Check sheet for the modelled part. Datum: model origin and axes. Units: mm. A direction names the side the tool comes from. Round coordinates to 2 decimals unless told otherwise and drop trailing zeros. Order: outer loops, then holes, each group sorted by start corner. A loop starts at its lowest first (then second) coordinate and runs counter-clockwise, first axis right, second up.
Q1. Set-up check for faces 1 (the flat face through (140, 20, -29.5)), 2 (the flat face through (66.49, 8.03, -16.82)), 3 (the flat face through (66.04, 12.08, -16.82)): record each of +Z, -Z, +X, -X, +Y, -Y from which the full face is reachable in a straight line by a thin tool's end or side.
Q2. Cross-section at A-A on x = 16.5. Record the cut outline in (y, z), then the cut area to 3 significant figures.
Q3. Depth check by flat-ended pin: P1, Ø8, axis at x = 133, y = 16, coming from the +Z side; P2, Ø10, axis at x = 160.5, z = -3.5, coming from the -Y side; P3, Ø4.5, axis at x = 246.5, z = -17, coming from the -Y side; P4, Ø3, axis at x = 235.5, z = -4, coming from the +Y side. Enter the tip coordinate at first touch or a pass-through.
Q4. Mould release check, pull along Z, two halves, no side actions. Record for faces 4 (the flat face through (250, 5, -34)), 5 (the cylindrical face through (16.6, 3.5, -19.5)), 6 (the flat face through (214.4, 11.944, -16.825)): +Z half, -Z half, draft (parallel to the pull), parting line (faces both ways), or undercut.
Q5. Cross-section at B-B on x = 213. Record the cut outline in (y, z).
Q6. Scan lines: probe 1 along X at (y, z) = (1.5, -17); probe 2 along X at (y, z) = (3, -16); probe 3 along Y at (x, z) = (18.5, -9.5). Record each from-to range of solid material in increasing order.
from build123d import *

# Parameters (mm, degrees)
SKETCH1_W             = 50
SKETCH1_H             = 34
BOSS_EXTRUDE1_DEPTH   = 10
BOSS_EXTRUDE1_2_DEPTH = 10
FILLET1_R             = 10
FILLET2_R             = 10
BOSS_EXTRUDE2_DEPTH   = 12.5
SKETCH4_R             = 2.5
CUT_EXTRUDE1_DEPTH    = 283.391465155
CHAMFER1_SIZE         = 3


with BuildPart() as part:
    # Sketch1 → Boss-Extrude1 (new body)
    with BuildSketch(Plane(origin=(0, 0, 0), x_dir=(1, 0, 0), z_dir=(0, 1, 0))):
        with Locations((25, 17)):
            Rectangle(SKETCH1_W, SKETCH1_H)
    extrude(amount=BOSS_EXTRUDE1_DEPTH)

    # Fillet1
    fillet1_edges = [part.edges().sort_by_distance(p)[0] for p in [
        (0, 5, -34),
        (0, 5, 0),
    ]]
    fillet(fillet1_edges, radius=FILLET1_R)



with BuildPart() as body_2:
    # Sketch1 → Boss-Extrude1 2 (new body)
    with BuildSketch(Plane(origin=(0, 0, 0), x_dir=(1, 0, 0), z_dir=(0, 1, 0))):
        with Locations((255, 17)):
            Rectangle(SKETCH1_W, SKETCH1_H)
    extrude(amount=BOSS_EXTRUDE1_2_DEPTH)

    # Fillet2
    fillet2_edges = [body_2.edges().sort_by_distance(p)[0] for p in [
        (280, 5, -34),
        (280, 5, 0),
    ]]
    fillet(fillet2_edges, radius=FILLET2_R)


with BuildPart() as part_1:
    add(part.part)

    add(body_2.part)  # Boss-Extrude2 merges body 2
    # Sketch3 → Boss-Extrude2 (add, symmetric)
    with BuildSketch(Plane.XY.offset(-17)):
        with BuildLine():
            Line((230, 7.094420761), (198.356689293, 16.93185641))
            add(Edge.make_bspline(
                [(198.356689293, 16.93185641), (197.921485468, 17.06715482), (197.058320029, 17.327430882), (195.247018989, 17.842283694), (192.878899734, 18.458259291), (189.862315722, 19.156901641), (185.625111362, 20.030310935), (179.946744848, 21.009637357), (172.608544526, 21.991371788), (164.84084187, 22.767908957), (154.046889349, 23.517083016), (140, 23.897827649), (125.953110651, 23.517083016), (115.15915813, 22.767908957), (107.391455474, 21.991371788), (100.053255152, 21.009637357), (94.374888638, 20.030310935), (90.137684278, 19.156901641), (87.121100266, 18.458259291), (84.752981011, 17.842283694), (82.941679971, 17.327430882), (82.078514532, 17.06715482), (81.643310707, 16.93185641)],
                knots=[0.641614074, 0.641614074, 0.641614074, 0.641614074, 0.67065102, 0.699687965, 0.757761856, 0.815835747, 0.873909637, 0.990057419, 1.106205201, 1.222352982, 1.338500764, 1.570796327, 1.80309189, 1.919239671, 2.035387453, 2.151535235, 2.267683016, 2.325756907, 2.383830798, 2.441904688, 2.470941634, 2.499978579, 2.499978579, 2.499978579, 2.499978579], degree=3))
            Line((81.643310707, 16.93185641), (50, 7.094420761))
            Line((50, 7.094420761), (50, 3.090164081))
            Line((50, 3.090164081), (50.593739641, 3.090164081))
            Line((50.593739641, 3.090164081), (82.83078999, 13.112184572))
            add(Edge.make_bspline(
                [(197.16921001, 13.112184572), (196.755159459, 13.240906743), (195.935388877, 13.488101862), (194.203464644, 13.980443227), (191.927236958, 14.572619906), (189.009827951, 15.248400933), (184.89320594, 16.097058438), (179.347389143, 17.053860827), (172.148362972, 18.017197671), (164.506098732, 18.781331097), (153.867128529, 19.519872284), (140, 19.895968137), (126.132871471, 19.519872284), (115.493901268, 18.781331097), (107.851637028, 18.017197671), (100.652610857, 17.053860827), (95.10679406, 16.097058438), (90.990172049, 15.248400933), (88.072763042, 14.572619906), (85.796535356, 13.980443227), (84.064611123, 13.488101862), (83.244840541, 13.240906743), (82.83078999, 13.112184572)],
                knots=[0.641614074, 0.641614074, 0.641614074, 0.641614074, 0.67065102, 0.699687965, 0.757761856, 0.815835747, 0.873909637, 0.990057419, 1.106205201, 1.222352982, 1.338500764, 1.570796327, 1.80309189, 1.919239671, 2.035387453, 2.151535235, 2.267683016, 2.325756907, 2.383830798, 2.441904688, 2.470941634, 2.499978579, 2.499978579, 2.499978579, 2.499978579], degree=3))
            Line((197.16921001, 13.112184572), (229.406260359, 3.090164081))
            Line((229.406260359, 3.090164081), (230, 3.090164081))
            Line((230, 3.090164081), (230, 7.094420761))
        make_face()
    extrude(amount=BOSS_EXTRUDE2_DEPTH, both=True)

    # Sketch4 → Cut-Extrude1 (cut, through all)
    with BuildSketch(Plane(origin=(0, 10, 0), x_dir=(1, 0, 0), z_dir=(0, 1, 0))):
        with Locations(Location((16.5, 17, 0), (0, 0, 270))):
            Circle(SKETCH4_R)
        with Locations(Location((33.5, 17, 0), (0, 0, 270))):
            Circle(SKETCH4_R)
        with Locations(Location((246.5, 17, 0), (0, 0, 270))):
            Circle(SKETCH4_R)
        with Locations(Location((263.5, 17, 0), (0, 0, 270))):
            Circle(SKETCH4_R)
    extrude(amount=-CUT_EXTRUDE1_DEPTH, mode=Mode.SUBTRACT)

    # Chamfer1
    chamfer1_edges = [part_1.edges().sort_by_distance(p)[0] for p in [
        (16.5, 10, -19.5),
        (33.5, 10, -19.5),
        (246.5, 10, -19.5),
        (263.5, 10, -19.5),
    ]]
    chamfer(chamfer1_edges, length=CHAMFER1_SIZE)


solid = part_1.part
Results found:
1. face 1: -Z, +Y, -Y
1. face 2: +Z, -Z, -Y
1. face 3: +Z, -Z, +Y
2. outline: (0, -34) - (10, -34) - (10, -22.5) - (7, -19.5) - (0, -19.5) - close; (0, -14.5) - (7, -14.5) - (10, -11.5) - (10, 0) - (0, 0) - close
2. area: 281 mm2
3. P1: stops at z = -4.5
3. P2: stops at y = 18.66
3. P3: passes through
3. P4: stops at y = 10
4. face 4: -Z half
4. face 5: undercut
4. face 6: draft
5. outline: (8.19, -29.5) - (12.38, -29.5) - (12.38, -4.5) - (8.19, -4.5) - close
6. probe 1: x = 0 to 14, 19 to 31, 36 to 50, 230 to 244, 249 to 261, 266 to 280
6. probe 2: x = 0 to 14.21, 18.79 to 31.21, 35.79 to 50, 230 to 244.21, 248.79 to 261.21, 265.79 to 280
6. probe 3: y = 0 to 10
